Check sheet for the drawn part. Datum: minimum x, y, z corner. Units: mm. Give positions to 0.01 mm unless a question says otherwise; leave off trailing zeros. Loops run counter-clockwise (first coordinate to the right, second up) from the corner with the lowest first, then second, coordinate; pieces in that order, holes last.
1. Cross-section at C-C, the plane y = 5. Record the cut outline in (x, z).
2. Go/stop test with a flat-tipped pin: pin 1 Ø6 at (x, y) = (10.5, 19) entering from -Z. Record where the tip stops, or that it passes through.
3. Cross-section at B-B, the plane x = 21.5. Record the cut outline in (y, z), plus the area to 3 significant figures.
4. Cross-section at A-A, the plane z = 14. Record the cut outline in (x, y), plus the area to 3 significant figures.
5. Material ranges on L1, parallel to X at y = 11.25, z = 14; L2, parallel to X at y = 12.5, z = 15; L3, parallel to Z at x = 21, y = 19, recorded low to high.
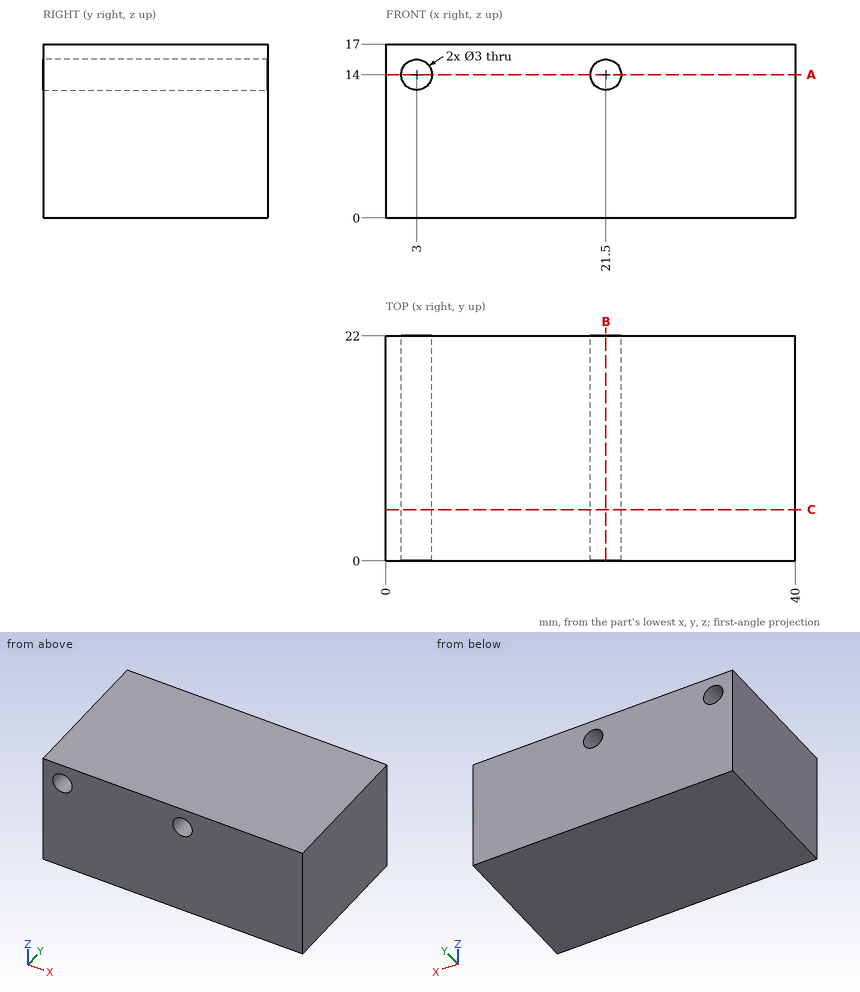
Result:
1. outline: (0, 0) - (40, 0) - (40, 17) - (0, 17) - close; hole circle Ø3 at (3, 14); hole circle Ø3 at (21.5, 14)
2. pin 1: stops at z = 0
3. outline: (0, 0) - (22, 0) - (22, 12.5) - (0, 12.5) - close; (0, 15.5) - (22, 15.5) - (22, 17) - (0, 17) - close
3. area: 308 mm2
4. outline: (0, 0) - (1.5, 0) - (1.5, 22) - (0, 22) - close; (4.5, 0) - (20, 0) - (20, 22) - (4.5, 22) - close; (23, 0) - (40, 0) - (40, 22) - (23, 22) - close
4. area: 748 mm2
5. L1: x = 0 to 1.5, 4.5 to 20, 23 to 40
5. L2: x = 0 to 1.88, 4.12 to 20.38, 22.62 to 40
5. L3: z = 0 to 12.59, 15.41 to 17
